Can you work these out from the drawing? Everything is in mm from the part's minimum corner. Coordinates: 2 decimals unless noted, no trailing zeros. Loops run counter-clockwise (first coordinate to the right, second up) from the corner with the lowest first, then second, coordinate; pieces in that order, holes last. Notation, with made-up numbers: M 72.5,66 L 128.5,66 A10 ccw 128.5,73 Z; hole C -33.5,82 d1. An arc over 180 degrees is marked long. Write each question's results on one line, items separated by ' | '.
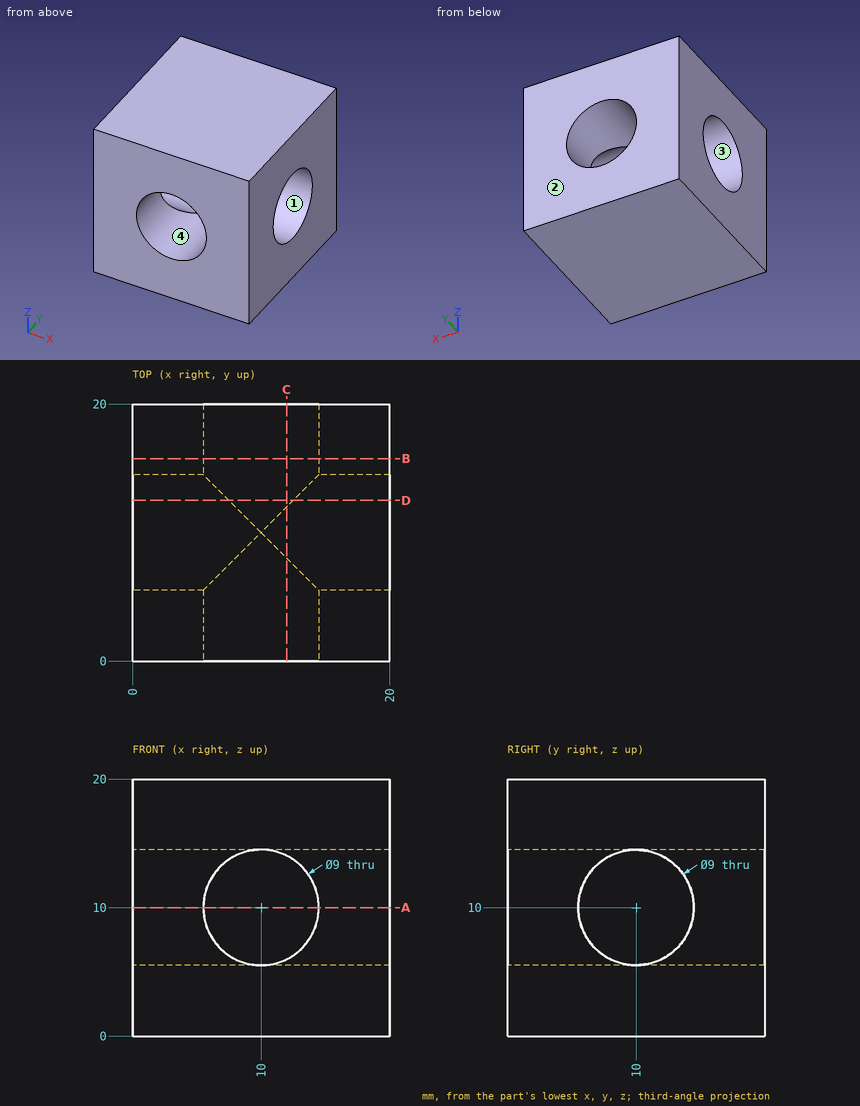
(1) Please list where this line runs through material, in increasing order: probe 1 along Z at (x, y) = (4, 10). Write a range as from..to.
Reported:
probe 1: z = 0..5.5, 14.5..20
(2) Imagine slicing it at B-B, the plane y = 15.75. List the corners of the cut face in (x, z) for me.
Reported:
outline: M 0,0 L 20,0 L 20,20 L 0,20 Z; hole C 10,10 d9
(3) Will these pins go through, and if not, where does the flat tip stop? P1, Ø1.5, axis at x = 10.5, y = 13, coming from the -Z side; P2, Ø8, axis at x = 10, z = 10, coming from the +Y side.
Reported:
P1: stops at z = 0 | P2: passes through
(4) If we mould it in two halves opening along Y, with no side actions, what happens to the marked faces 1, 2, 3 and 4? For each: released by +Y, released by -Y, zero draft, split by the parting line, or undercut.
Reported:
face 1: undercut | face 2: released by +Y | face 3: undercut | face 4: zero draft
(5) Imagine slicing it at C-C, the plane x = 12. List the corners of the cut face in (y, z) for me.
Reported:
outline: M 0,0 L 20,0 L 20,5.97 L 12,5.97 A4.5 cw 8,5.97 L 0,5.97 Z; M 0,14.03 L 8,14.03 A4.5 cw 12,14.03 L 20,14.03 L 20,20 L 0,20 Z
(6) Imagine slicing it at A-A, the plane z = 10. List the corners of the cut face in (x, y) for me.
Reported:
outline: M 0,0 L 5.5,0 L 5.5,5.5 L 0,5.5 Z; M 0,14.5 L 5.5,14.5 L 5.5,20 L 0,20 Z; M 14.5,0 L 20,0 L 20,5.5 L 14.5,5.5 Z; M 14.5,14.5 L 20,14.5 L 20,20 L 14.5,20 Z
(7) Imagine slicing it at D-D, the plane y = 12.5. List the corners of the cut face in (x, z) for me.
Reported:
outline: M 0,0 L 20,0 L 20,6.26 L 12.5,6.26 A4.5 cw 7.5,6.26 L 0,6.26 Z; M 0,13.74 L 7.5,13.74 A4.5 cw 12.5,13.74 L 20,13.74 L 20,20 L 0,20 Z
